from build123d import *

# Parameters (mm, degrees)
SKETCH1_W           = 114
SKETCH1_H           = 114
SKETCH1_W_2         = 110
SKETCH1_H_2         = 110
BOSS_EXTRUDE1_DEPTH = 2
SKETCH1_3_W         = 114
SKETCH1_3_H         = 114
SKETCH1_3_W_2       = 110
SKETCH1_3_H_2       = 110
BOSS_EXTRUDE2_DEPTH = 40
SKETCH2_W           = 48.37766652
SKETCH2_H           = 27.964547649
SKETCH2_W_2         = 49.350090125
SKETCH2_H_2         = 19.287013153
CUT_EXTRUDE1_DEPTH  = 132.882523482
FILLET1_R           = 5
FILLET2_R           = 5


with BuildPart() as part:
    # Sketch1 → Boss-Extrude1 (new body)
    # profile 1 of 2: a face of its own
    with BuildSketch(Plane(origin=(0, 0, 0), x_dir=(1, 0, 0), z_dir=(0, 1, 0))):
        Rectangle(SKETCH1_W, SKETCH1_H)
        Rectangle(SKETCH1_W_2, SKETCH1_H_2, mode=Mode.SUBTRACT)
    # profile 2 of 2: a face of its own
    with BuildSketch(Plane(origin=(0, 0, 0), x_dir=(1, 0, 0), z_dir=(0, 1, 0))):
        Rectangle(SKETCH1_W_2, SKETCH1_H_2)
    extrude(amount=BOSS_EXTRUDE1_DEPTH)

    # Sketch1<3> → Boss-Extrude2 (add)
    with BuildSketch(Plane(origin=(0, 0, 0), x_dir=(1, 0, 0), z_dir=(0, 1, 0))):
        Rectangle(SKETCH1_3_W, SKETCH1_3_H)
        Rectangle(SKETCH1_3_W_2, SKETCH1_3_H_2, mode=Mode.SUBTRACT)
    extrude(amount=BOSS_EXTRUDE2_DEPTH)

    # Sketch2 → Cut-Extrude1 (cut, through all)
    with BuildSketch(Plane.XY.offset(-55)):
        with Locations((30.81116674, 15.982273825)):
            Rectangle(SKETCH2_W, SKETCH2_H)
        with Locations((-30.324954937, 11.643506577)):
            Rectangle(SKETCH2_W_2, SKETCH2_H_2)
    extrude(amount=-CUT_EXTRUDE1_DEPTH, mode=Mode.SUBTRACT)

    # Fillet1
    # the kernel refuses this fillet: 5 mm, written as the material it adds along each edge
    with BuildSketch(Plane(origin=(50, 7, 50), x_dir=(0, 0, 1), z_dir=(0, -1, 0))) as fillet1_piece_1_section:
        Polygon((0, 0), (FILLET1_R, 0), (FILLET1_R, -FILLET1_R), (0, -FILLET1_R), align=None)
    fillet1_piece_1 = extrude(amount=FILLET1_R, mode=Mode.PRIVATE)
    fillet1_piece_1 = fillet1_piece_1 - Plane(origin=(50, 7, 50), x_dir=(-0.7071067811865477, 0, -0.7071067811865475), z_dir=(0, -1, 0)) * Sphere(FILLET1_R, mode=Mode.PRIVATE)
    add(fillet1_piece_1)
    with BuildSketch(Plane(origin=(-50, 7, 50), x_dir=(-1, 0, 0), z_dir=(0, -1, 0))) as fillet1_piece_2_section:
        Polygon((0, 0), (FILLET1_R, 0), (FILLET1_R, -FILLET1_R), (0, -FILLET1_R), align=None)
    fillet1_piece_2 = extrude(amount=FILLET1_R, mode=Mode.PRIVATE)
    fillet1_piece_2 = fillet1_piece_2 - Plane(origin=(-50, 7, 50), x_dir=(0.7071067811865475, 0, -0.7071067811865476), z_dir=(0, -1, 0)) * Sphere(FILLET1_R, mode=Mode.PRIVATE)
    add(fillet1_piece_2)
    with BuildSketch(Plane(origin=(55, 2, 50), x_dir=(0, 1, 0), z_dir=(0, 0, -1)), Plane(origin=(-55, 2, -57), x_dir=(0, 1, 0), z_dir=(0, 0, 1))) as fillet1_piece_3:
        with BuildLine():
            CenterArc((FILLET1_R, -FILLET1_R), FILLET1_R, 90, 90)
            Line((0, -FILLET1_R), (0, 0))
            Line((0, 0), (FILLET1_R, 0))
        make_face()
    extrude(amount=107)
    with BuildSketch(Plane(origin=(50, 2, 55), x_dir=(0, 1, 0), z_dir=(-1, 0, 0))) as fillet1_piece_4:
        with BuildLine():
            CenterArc((FILLET1_R, FILLET1_R), FILLET1_R, 180, 90)
            Line((0, FILLET1_R), (0, 0))
            Line((0, 0), (FILLET1_R, 0))
        make_face()
    extrude(amount=100)
    with BuildSketch(Plane(origin=(-55, 7, 55), x_dir=(0, 0, -1), z_dir=(0, 1, 0)), Plane(origin=(55, 7, 55), x_dir=(-1, 0, 0), z_dir=(0, 1, 0))) as fillet1_piece_5:
        with BuildLine():
            CenterArc((FILLET1_R, -FILLET1_R), FILLET1_R, 90, 90)
            Line((0, -FILLET1_R), (0, 0))
            Line((0, 0), (FILLET1_R, 0))
        make_face()
    extrude(amount=33)
    with BuildSketch(Plane(origin=(55, 29.964547649, -55), x_dir=(-1, 0, 0), z_dir=(0, 1, 0))) as fillet1_piece_6:
        with BuildLine():
            CenterArc((FILLET1_R, FILLET1_R), FILLET1_R, 180, 90)
            Line((0, FILLET1_R), (0, 0))
            Line((0, 0), (FILLET1_R, 0))
        make_face()
    extrude(amount=10.035452351)
    with BuildSketch(Plane(origin=(-55, 21.287013153, -55), x_dir=(1, 0, 0), z_dir=(0, 1, 0))) as fillet1_piece_7:
        with BuildLine():
            CenterArc((FILLET1_R, -FILLET1_R), FILLET1_R, 90, 90)
            Line((0, -FILLET1_R), (0, 0))
            Line((0, 0), (FILLET1_R, 0))
        make_face()
    extrude(amount=18.712986847)
    # the kernel refuses this fillet: 5 mm, written as the material it takes off along each edge
    with BuildSketch(Plane(origin=(69.5, 0, 57), x_dir=(0, 0, -1), z_dir=(-1, 0, 0))) as fillet1_2_piece_1:
        with BuildLine():
            CenterArc((FILLET1_R, -FILLET1_R), FILLET1_R, 90, 90)
            Line((0, -FILLET1_R), (0, 0))
            Line((0, 0), (FILLET1_R, 0))
        make_face()
    extrude(amount=139, mode=Mode.SUBTRACT)
    with BuildSketch(Plane(origin=(-57, -12.5, 57), x_dir=(1, 0, 0), z_dir=(0, 1, 0)), Plane(origin=(57, 52.5, 57), x_dir=(-1, 0, 0), z_dir=(0, -1, 0))) as fillet1_2_piece_2:
        with BuildLine():
            CenterArc((FILLET1_R, FILLET1_R), FILLET1_R, 180, 90)
            Line((0, FILLET1_R), (0, 0))
            Line((0, 0), (FILLET1_R, 0))
        make_face()
    extrude(amount=65, mode=Mode.SUBTRACT)
    with BuildSketch(Plane(origin=(57, 52.5, -57), x_dir=(-1, 0, 0), z_dir=(0, -1, 0)), Plane(origin=(-57, -12.5, -57), x_dir=(1, 0, 0), z_dir=(0, 1, 0))) as fillet1_2_piece_3:
        with BuildLine():
            CenterArc((FILLET1_R, -FILLET1_R), FILLET1_R, 90, 90)
            Line((0, -FILLET1_R), (0, 0))
            Line((0, 0), (FILLET1_R, 0))
        make_face()
    extrude(amount=65, mode=Mode.SUBTRACT)

    # Fillet2
    # the kernel refuses this fillet: 5 mm, written as the material it takes off along each edge
    with BuildSketch(Plane(origin=(52, 5, 52), x_dir=(0, -1, 0), z_dir=(1, 0, 0))) as fillet2_piece_1_section:
        Polygon((0, 0), (FILLET2_R, 0), (FILLET2_R, -FILLET2_R), (0, -FILLET2_R), align=None)
    fillet2_piece_1 = extrude(amount=FILLET2_R, mode=Mode.PRIVATE)
    fillet2_piece_1 = fillet2_piece_1 - Plane(origin=(52, 5, 52), x_dir=(0, 0.7071067811865475, -0.7071067811865475), z_dir=(1, 0, 0)) * Sphere(FILLET2_R, mode=Mode.PRIVATE)
    add(fillet2_piece_1, mode=Mode.SUBTRACT)
    with BuildSketch(Plane(origin=(-52, 5, 52), x_dir=(0, -1, 0), z_dir=(-1, 0, 0))) as fillet2_piece_2_section:
        Polygon((0, 0), (FILLET2_R, 0), (FILLET2_R, FILLET2_R), (0, FILLET2_R), align=None)
    fillet2_piece_2 = extrude(amount=FILLET2_R, mode=Mode.PRIVATE)
    fillet2_piece_2 = fillet2_piece_2 - Plane(origin=(-52, 5, 52), x_dir=(0, 0.7071067811865475, -0.7071067811865475), z_dir=(-1, 0, 0)) * Sphere(FILLET2_R, mode=Mode.PRIVATE)
    add(fillet2_piece_2, mode=Mode.SUBTRACT)
    with BuildSketch(Plane(origin=(57, 0, -52), x_dir=(0, 1, 0), z_dir=(0, 0, 1)), Plane(origin=(-52, 0, -57), x_dir=(0, 1, 0), z_dir=(1, 0, 0)), Plane(origin=(-57, 0, 52), x_dir=(0, 1, 0), z_dir=(0, 0, -1))) as fillet2_piece_3:
        with BuildLine():
            CenterArc((FILLET2_R, FILLET2_R), FILLET2_R, 180, 90)
            Line((0, FILLET2_R), (0, 0))
            Line((0, 0), (FILLET2_R, 0))
        make_face()
    extrude(amount=104, mode=Mode.SUBTRACT)
    with BuildSketch(Plane(origin=(52, 0, -52), x_dir=(1, 0, 0), z_dir=(0, 0, 1))) as fillet2_piece_4:
        with BuildLine():
            CenterArc((5 - FILLET2_R, FILLET2_R), FILLET2_R, 270, 90)
            Line((5 - FILLET2_R, 0), (5, 0))
            Line((5, 0), (5, FILLET2_R))
        make_face()
    revolve(axis=Axis((52, 0, -52), (0, 1, 0)), revolution_arc=90, mode=Mode.SUBTRACT)
    with BuildSketch(Plane(origin=(-52, 0, -52), x_dir=(-1, 0, 0), z_dir=(0, 0, 1))) as fillet2_piece_5:
        with BuildLine():
            CenterArc((5 - FILLET2_R, -FILLET2_R), FILLET2_R, 0, 90)
            Line((5 - FILLET2_R, 0), (5, 0))
            Line((5, 0), (5, -FILLET2_R))
        make_face()
    revolve(axis=Axis((-52, 0, -52), (0, -1, 0)), revolution_arc=90, mode=Mode.SUBTRACT)


solid = part.part
Source: CAD feature listing. Evaluate the final solid. Frame: model axes, mm. A direction names the side the tool comes from. Round coordinates to 2 decimals unless told otherwise and drop trailing zeros. Loops run counter-clockwise (first coordinate to the right, second up) from the corner with the lowest first, then second, coordinate; pieces in that order, holes last.
Q1. First-contact query: P1, Ø1, axis at x = 30.5, y = 24, coming from the -Z side; P2, Ø1.6, axis at y = 10, z = -56.5, coming from the +X side; P3, Ø3.5, axis at x = 35, z = -54, coming from the -Y side. Flat tips, straight axial feed; report the tip coordinate or a pass-through.
Q2. Section A-A, the plane y = 13. Return loops of the section in (x, z), plus the area to 3 significant figures.
Q3. Mould query, pull axis Y, two halves, no side actions, for faces 4 (the face through (57, 22, 1)), 5 (the face through (-55, 1, 1)), 6 (the face through (31, 29.965, -56)). Classes: pulls with the +Y half, pulls with the -Y half, needs draft (parallel to the pull), parting line crosses it, or undercut.
Q4. Section D-D, the plane y = 31.5. Return loops of the section in (x, z), plus the area to 3 significant figures.
Q5. Section C-C, the plane z = -41.5. Return loops of the section in (x, y), plus the area to 3 significant figures.
Q6. Access query for faces 1 (the face through (-56, 26, -55)), 2 (the face through (-30, 21.287, -56)), 3 (the face through (-53, 31, -54)). Directions: +Z, -Z, +X, -X, +Y, -Y. A direction counts if a zero-diameter tool reaches every point of the face in a straight line with its end or side. Return the directions, or none.
Q7. Section B-B, the plane x = 41.5. Return loops of the section in (y, z), plus the area to 3 significant figures.
Q8. Ray query, line 1 (X direction, y = 32, z = -10); line 2 (Y direction, x = -38, z = -1.5). Return the intervals inside material, ascending.
Solutions:
1. P1: stops at z = 55
1. P2: stops at x = 55.36
1. P3: stops at y = 0.01
2. outline: (-57, -52) arc R5 ccw to (-55, -56) - (-55, 50) arc R5 cw to (-50, 55) - (50, 55) arc R5 cw to (55, 50) - (55, -56) arc R5 ccw to (57, -52) - (57, 52) arc R5 ccw to (52, 57) - (-52, 57) arc R5 ccw to (-57, 52) - close; (-5.65, -57) - (6.62, -57) - (6.62, -55) - (-5.65, -55) - close
2. area: 692 mm2
3. face 4: needs draft
3. face 5: pulls with the -Y half
3. face 6: undercut
4. outline: (-57, -52) arc R5 ccw to (-52, -57) - (52, -57) arc R5 ccw to (57, -52) - (57, 52) arc R5 ccw to (52, 57) - (-52, 57) arc R5 ccw to (-57, 52) - close; hole (-55, -50) arc R5 ccw to (-50, -55) - (50, -55) arc R5 ccw to (55, -50) - (55, 50) arc R5 ccw to (50, 55) - (-50, 55) arc R5 ccw to (-55, 50) - close
4. area: 896 mm2
5. outline: (-57, 5) arc R5 ccw to (-52, 0) - (52, 0) arc R5 ccw to (57, 5) - (57, 40) - (55, 40) - (55, 7) arc R5 cw to (50, 2) - (-50, 2) arc R5 cw to (-55, 7) - (-55, 40) - (-57, 40) - close
5. area: 380 mm2
6. face 1: -Z, -X, +Y, -Y
6. face 2: -Z
6. face 3: +Y
7. outline: (0, -52) arc R5 ccw to (2, -56) - (2, 50) arc R5 cw to (7, 55) - (40, 55) - (40, 57) - (5, 57) arc R5 ccw to (0, 52) - close; (29.96, -57) - (40, -57) - (40, -55) - (29.96, -55) - close
7. area: 320 mm2
8. line 1: x = -57 to -55, 55 to 57
8. line 2: y = 0 to 2
